The listing builds one solid part. Answer for the finished solid, in the listing's coordinates (mm). A direction names the side the tool comes from. Give positions to 0.01 mm unless a question says otherwise; leave off trailing zeros. Order: outer loops, then holes, each group sorted by start corner. A loop starts at its lowest first (then second) coordinate and runs counter-clockwise, first axis right, second up. Notation, with made-up numbers: M 85,48 L 107,48 A29 ccw 107,69 Z; hole C -4.75,-40 d11. An arc over 180 degrees is marked long. Answer as a JSON object with one key per item and string values. Group by question number.
```python
from build123d import *

# Parameters (mm, degrees)
F_0015_CYLINDER_SKETCH_R    = 3.25
F_0015_CYLINDER_DEPTH       = 2.5
F_0016_FILLET_R             = 0.625
F_0017_EXTRUDE_DEPTH        = 1.385
F_0017_EXTRUDE_ROTATE_ANGLE = 120
F_0020_CYLINDER_SKETCH_R    = 1.2
F_0020_CYLINDER_DEPTH       = 9.7
F_0021_CONE_ROTATE_ANGLE    = 90


with BuildPart() as part:
    # 0015_cylinder_Sketch → 0015_cylinder (new body)
    with BuildSketch(Plane.XY):
        Circle(F_0015_CYLINDER_SKETCH_R)
    extrude(amount=F_0015_CYLINDER_DEPTH)

    # 0016_fillet
    f_0016_fillet_edges = [part.edges().sort_by_distance(p)[0] for p in [
        (-3.25, 0, 2.5),
    ]]
    fillet(f_0016_fillet_edges, radius=F_0016_FILLET_R)


with BuildPart() as body_2:
    # 0017_extrude_Sketch → 0017_extrude (new body)
    with BuildSketch(Plane.XY):
        Polygon((0, 0), (1.154700538, 0), (1.732050808, 1), (1.154700538, 2), (0, 2), (-0.577350269, 1), align=None)
    extrude(amount=F_0017_EXTRUDE_DEPTH)


with BuildPart() as body_2_1:
    # 0017_extrude_Rotate: read off the stored shape, not the designer's step
    # 0017_extrude_Rotate: moved
    add(body_2.part.rotate(Axis((0, 0, 0), (0, 0, 1)), F_0017_EXTRUDE_ROTATE_ANGLE))


with BuildPart() as body_2_2:
    # 0017_extrude_Translate: moved
    add(body_2_1.part.moved(Location((1.154700538, 0, 1.125))))


with BuildPart() as part_1:
    add(part.part)

    # 0019_sub: cut body 2
    add(body_2_2.part, mode=Mode.SUBTRACT)


with BuildPart() as body_2_2_1:
    # 0020_cylinder_Sketch → 0020_cylinder (new body)
    with BuildSketch(Plane.XY):
        Circle(F_0020_CYLINDER_SKETCH_R)
    extrude(amount=F_0020_CYLINDER_DEPTH)


with BuildPart() as body_2_2_2:
    # 0020_cylinder_Translate: moved
    add(body_2_2_1.part.moved(Location((0, 0, -9.7))))


with BuildPart() as body_3:
    # 0021_cone_Sketch → 0021_cone (revolve)
    with BuildSketch(Plane.XY, mode=Mode.PRIVATE) as f_0021_cone_sk:
        Polygon((0, 0), (1.2, 0), (0.9, 0.3), (0, 0.3), align=None)
    revolve(f_0021_cone_sk.sketch.rotate(Axis((0, -100, 0), (0, 1, 0)), 90), axis=Axis((0, -100, 0), (0, 1, 0)))


with BuildPart() as body_3_1:
    # 0021_cone_Rotate: moved
    add(body_3.part.rotate(Axis((0, 0, 0), (1, 0, 0)), F_0021_CONE_ROTATE_ANGLE))


with BuildPart() as body_3_2:
    # 0021_cone_Translate: moved
    add(body_3_1.part.moved(Location((0, 0, -10))))


with BuildPart() as body_2_2_3:
    add(body_2_2_2.part)

    # 0023_add: union body 3
    add(body_3_2.part)


with BuildPart() as part_2:
    add(part_1.part)

    # 0024_add: union body 2 2
    add(body_2_2_3.part)


solid = part_2.part
```
Item 1: Determine the mould class of faces 4 (the flat face through (1, -1, 2.5)), 5 (the flat face through (0, -1, 2)), 6 (the cylindrical face through (0.65, 1.01, -4.92)) for opening direction Y: released by +Y, released by -Y, zero draft, split by the parting line, or undercut.
Item 2: A tool of negligible diameter and unlimited length cuts with its end or side. For faces 1 (the flat face through (0, 1, 2)), 2 (the flat face through (1.4, 0, 0)), 3 (the flat face through (0, 0, -10)), from which of +Z, -Z, +X, -X, +Y, -Y can it reach the whole face along a straight path? Write none if from no direction.
Item 3: Section C-C (z = -6) is taken. Determine the outline of the cut face in (x, y).
Item 4: Flat-ended cylindrical pins translate along their axes: P1, Ø1.5, axis at x = -2, y = 1.5, coming from the -Z side; P2, Ø2, axis at y = -1.5, z = -5.5, coming from the -X side; P3, Ø3, axis at x = 0, z = -3, coming from the -Y side. Find the tip coordinate at first contact, or state that the pin passes through.
Item 5: Consider probe 1 along Z at (x, y) = (1.25, 1.5); probe 2 along Y at (x, z) = (0, -3.5); probe 3 along Z at (x, y) = (0.5, 0.5) (3 decimals). Determine where each line is inside the solid, lowest interval first. Write a range as from..to.
Item 6: Section A-A (z = 1.25) is taken. Determine the outline of the cut face in (x, y), and give its area (3 significant figures).
Item 7: Section B-B (x = 0) is taken. Determine the outline of the cut face in (y, z) (3 decimals).
Values found:
{
 "1": {"face 4": "zero draft", "face 5": "undercut", "face 6": "split by the parting line"},
 "2": {"face 1": "+Z", "face 2": "-Z", "face 3": "-Z, +X, -X, +Y, -Y"},
 "3": {"outline": "C 0,0 d2.4"},
 "4": {"P1": "stops at z = 0", "P2": "stops at x = -1.09", "P3": "stops at y = -1.2"},
 "5": {"probe 1": "z = 0..2.5", "probe 2": "y = -1.2..1.2", "probe 3": "z = -10..1.125"},
 "6": {"outline": "C 0,0 d6.5; hole M -1.15,0 L -0.58,-1 L 0.58,-1 L 1.15,0 L 0.58,1 L -0.58,1 Z", "area": "29.7 mm^2"},
 "7": {"outline": "M -3.25,0 L -1.2,0 L -1.2,-9.7 L -0.9,-9.7 L -1.2,-10 L 1.2,-10 L 0.9,-9.7 L 1.2,-9.7 L 1.2,0 L 3.25,0 L 3.25,1.875 A0.625 ccw 2.625,2.5 L 1,2.5 L 1,1.125 L -1,1.125 L -1,2.5 L -2.625,2.5 A0.625 ccw -3.25,1.875 Z"}
}
